```python
from build123d import *

# Parameters (mm, degrees)
ESQUISSE1_R                = 5.9
BOSS_EXTRU_1_DEPTH         = 6.5
ESQUISSE2_R                = 1.25
ENL_V_MAT_EXTRU_1_DEPTH    = 1.5
R_P_TITION_LIN_AIRE1_COUNT = 2
R_P_TITION_LIN_AIRE1_PITCH = 7.3


with BuildPart() as part:
    # Esquisse1 → Boss.-Extru.1 (new body)
    with BuildSketch(Plane(origin=(0, 0, 0), x_dir=(1, 0, 0), z_dir=(0, 1, 0))):
        Circle(ESQUISSE1_R)
    extrude(amount=BOSS_EXTRU_1_DEPTH)

    # Esquisse2 → Enlèv. mat.-Extru.1 (cut)
    with BuildSketch(Plane(origin=(0, 6.5, 0), x_dir=(1, 0, 0), z_dir=(0, 1, 0))):
        Circle(ESQUISSE2_R)
    extrude(amount=-ENL_V_MAT_EXTRU_1_DEPTH, mode=Mode.SUBTRACT)

    # Esquisse4 → Révolution1 (revolve)
    with BuildSketch(Plane.XY):
        with BuildLine():
            Line((-3.65, -3), (-4.1, -3))
            Line((-4.1, -3), (-4.1, -2.2))
            ThreePointArc((-4.1, -2.2), (-4.26109127, -1.81109127), (-4.65, -1.65))
            Line((-4.65, -1.65), (-4.65, -1.6))
            Line((-4.65, -1.6), (-4.1, -1.6))
            Line((-4.1, -1.6), (-4.1, 0))
            Line((-4.1, 0), (-3.65, 0))
            Line((-3.65, 0), (-3.65, -3))
        make_face()
    r_volution1 = revolve(axis=Axis((-3.65, 0, 0), (0, -1, 0)))

    # Répétition linéaire1: Révolution1 ×2
    with Locations(*[(i * R_P_TITION_LIN_AIRE1_PITCH, 0, 0) for i in range(1, R_P_TITION_LIN_AIRE1_COUNT)]):
        add(r_volution1)


solid = part.part
```
For this review, take the finished solid that the model builds, in its own axes (mm). A direction names the side the tool comes from. Coordinates: 2 decimals unless noted, no trailing zeros. Write each loop counter-clockwise with the first axis right and the second up, starting at its lowest first coordinate (ties: lowest second). Pieces come first, ordered by that corner, then holes. Notation, with made-up numbers: (-13, -31.75) - (32, -31.75) arc R11 cw to (32, -10.75) - close; hole circle Ø2 at (-4.5, 56). An arc over 180 degrees is marked (long way). Answer in a Markdown table with one row per item. Add a question column.
Q1. For probe 1 along Z at (x, y) = (0, 5.5); probe 2 along Y at (x, z) = (-2.5, 2.5), list the stretches that pass through material, from the lowest coordinate up.
Q2. We need section B-B, the plane x = 0. State the section outline as (y, z) points, and give its area (4 significant figures).
Q3. We need section A-A, the plane y = -0.25. State the section outline as (x, z) points.
Q4. Tool access review of faces 1 (the cylindrical face through (-5.894, 3.204, -0.259)), 2 (the cylindrical face through (4.1, -2.6, 0)), 3 (the cylindrical face through (-4.079, -0.789, -0.135)), 4 (the flat face through (3.6, -3, 0)), 5 (the cylindrical face through (-0.27, 5.76, 1.22)): name each direction out of +Z, -Z, +X, -X, +Y, -Y from which nothing blocks a thin tool from reaching the whole face with its end or side.
Q5. We need section D-D, the plane x = 3.65. State the section outline as (y, z) points, and give its area (3 significant figures).
Q6. For P1, Ø5, axis at x = -2, y = 4, coming from the +Z side; P2, Ø5, axis at x = 4.5, y = 1, coming from the +Z side; P3, Ø6, axis at x = 1.5, z = 3, coming from the -Y side; P4, Ø2, axis at x = 2.5, y = 2, coming from the -Z side, all flat-tipped, find the tip position at first contact; note any pin that passes through.
Q7. Draft analysis for pull direction Y (two halves, no side actions). For faces 6 (the cylindrical face through (4.1, -0.8, 0)), 7 (the flat face through (-0.1, 6.5, -1.4)), 8 (the cylindrical face through (-4.079, -2.594, -0.135)), state which applies: +Y half, -Y half, draft (parallel to the pull), parting line (faces both ways), or undercut.
Answer list:
| question | item | result |
|---|---|---|
| 1 | probe 1 | z = -5.9 to -1.25, 1.25 to 5.9 |
| 1 | probe 2 | y = 0 to 6.5 |
| 2 | outline | (0, -5.9) - (6.5, -5.9) - (6.5, -1.25) - (5, -1.25) - (5, 1.25) - (6.5, 1.25) - (6.5, 5.9) - (0, 5.9) - close |
| 2 | area | 72.95 mm2 |
| 3 | outline | circle Ø0.9 at (-3.65, 0); circle Ø0.9 at (3.65, 0) |
| 4 | face 1 | +Y, -Y |
| 4 | face 2 | -Y |
| 4 | face 3 | none |
| 4 | face 4 | +Z, -Z, +X, -X, -Y |
| 4 | face 5 | +Y |
| 5 | outline | (-3, -0.45) - (-2.2, -0.45) arc R0.55 cw to (-1.65, -1) - (-1.6, -1) - (-1.6, -0.45) - (0, -0.45) - (0, -4.64) - (6.5, -4.64) - (6.5, 4.64) - (0, 4.64) - (0, 0.45) - (-1.6, 0.45) - (-1.6, 1) - (-1.65, 1) arc R0.55 cw to (-2.2, 0.45) - (-3, 0.45) - close |
| 5 | area | 63.1 mm2 |
| 6 | P1 | stops at z = 5.9 |
| 6 | P2 | stops at z = 5.55 |
| 6 | P3 | stops at y = -1.75 |
| 6 | P4 | stops at z = -5.71 |
| 7 | face 6 | undercut |
| 7 | face 7 | +Y half |
| 7 | face 8 | draft |
